Study the drawing (mm; zero at the part's minimum x, y, z) and answer. A direction names the side the tool comes from. Give positions to 0.01 mm unless a question says otherwise; leave off trailing zeros. Order: outer loops, then holes, each group sorted by start corner. A loop starts at its lowest first (then second) coordinate and runs counter-clockwise, first axis right, second up.
Item 1: A cutting plane is placed at B-B (x = 7). Write down the section's boundary in (y, z).
Item 2: A cutting plane is placed at D-D (y = 28). Write down the section's boundary in (x, z), plus the area to 3 significant figures.
Item 3: Find the intervals of material crossed by line 1 along X through (y, z) = (16.5, 8.75); line 2 along Y through (x, z) = (19.25, 7.25); line 3 along Z through (x, y) = (6.75, 11), in increasing order.
Item 4: A cutting plane is placed at C-C (z = 9.5). Write down the section's boundary in (x, y).
Item 5: Which of the six approach directions +Z, -Z, +X, -X, +Y, -Y give full straight-line access (tool end or side, diameter ignored) to the marked faces 1, 2 and 3?
Item 6: A cutting plane is placed at A-A (y = 18). Write down the section's boundary in (x, z).
Item 7: Given pin 1 Ø1.5 at (x, y) = (16.5, 8.5) entering from +Z; pin 2 Ø6 at (x, z) = (8, 10.5) entering from -Y; pin 3 Ø12 at (y, z) = (27, 13.5) entering from +X (1 decimal), each flat-ended and moving along its own axis, determine where each tip first touches the part or whether it passes through.
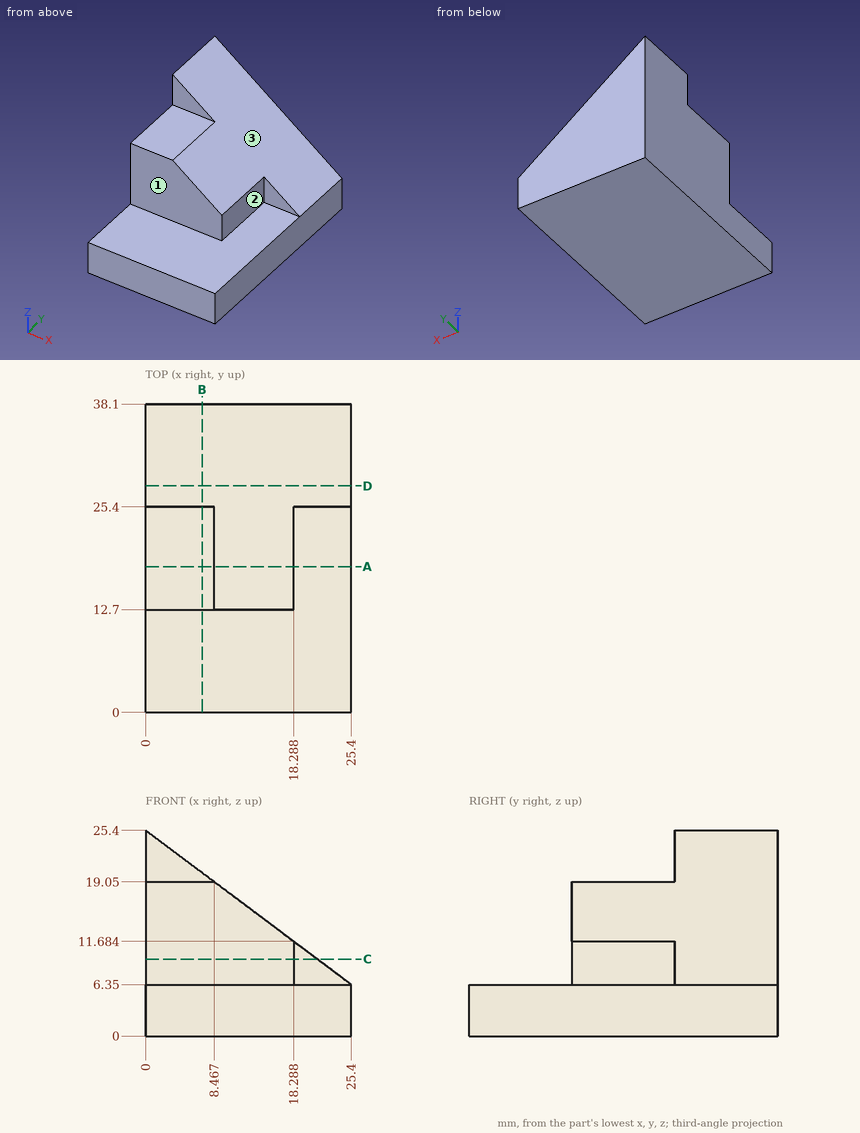
Response values:
1. outline: (0, 0) - (38.1, 0) - (38.1, 20.15) - (25.4, 20.15) - (25.4, 19.05) - (12.7, 19.05) - (12.7, 6.35) - (0, 6.35) - close
2. outline: (0, 0) - (25.4, 0) - (25.4, 6.35) - (0, 25.4) - close
2. area: 403 mm2
3. line 1: x = 0 to 18.29
3. line 2: y = 25.4 to 38.1
3. line 3: z = 0 to 6.35
4. outline: (0, 12.7) - (18.29, 12.7) - (18.29, 25.4) - (21.2, 25.4) - (21.2, 38.1) - (0, 38.1) - close
5. face 1: +Z, +X, -X, -Y
5. face 2: +Z, +X, -Y
5. face 3: +Z, +X, +Y, -Y
6. outline: (0, 0) - (25.4, 0) - (25.4, 6.35) - (18.29, 6.35) - (18.29, 11.68) - (8.47, 19.05) - (0, 19.05) - close
7. pin 1: stops at z = 6.35
7. pin 2: stops at y = 12.7
7. pin 3: stops at x = 23.9
